Autodesk Inventor part; units mm, degrees
ref_plane "YZ Plane" through (0, 0, 0) normal (1, 0, 0) x (0, 1, 0)
ref_plane "XZ Plane" through (0, 0, 0) normal (0, 1, 0) x (-1, 0, 0)
ref_plane "XY Plane" through (0, 0, 0) normal (0, 0, 1) x (1, 0, 0)
sketch "Sketch1" plane through (0, 0, 0) normal (0, 0, 1) x (1, 0, 0)
  line L0 (0, 0) -> (0, 20) construction
  line L1 (2.5, 15) -> (97.5, 15)
  line L2 (97.5, 15) -> (97.5, -15)
  line L3 (97.5, -15) -> (2.5, -15)
  line L4 (2.5, -15) -> (2.5, 15)
  line L5 (2.5, 15) -> (97.5, -15) construction
  line L6 (97.5, 15) -> (2.5, -15) construction
  line L7 (40, 5) -> (60, 5)
  line L8 (60, 5) -> (60, -5)
  line L9 (60, -5) -> (40, -5)
  line L10 (40, -5) -> (40, 5)
  line L11 (40, 5) -> (60, -5) construction
  line L12 (60, 5) -> (40, -5) construction
  line L13 (60, 5) -> (60, 15)
  line L14 (60, -5) -> (60, -15)
  line L15 (-2.5, 15) -> (-97.5, 15)
  line L16 (-97.5, 15) -> (-97.5, -15)
  line L17 (-97.5, -15) -> (-2.5, -15)
  line L18 (-2.5, -15) -> (-2.5, 15)
  line L19 (-2.5, 15) -> (-97.5, -15) construction
  line L20 (-97.5, 15) -> (-2.5, -15) construction
  line L21 (-40, 5) -> (-60, 5)
  line L22 (-60, 5) -> (-60, -5)
  line L23 (-60, -5) -> (-40, -5)
  line L24 (-40, -5) -> (-40, 5)
  line L25 (-40, 5) -> (-60, -5) construction
  line L26 (-60, 5) -> (-40, -5) construction
  line L27 (-60, 5) -> (-60, 15)
  line L28 (-60, -5) -> (-60, -15)
  line L29 (-45, 45) -> (45, 45)
  line L30 (45, 45) -> (45, -45)
  line L31 (45, -45) -> (-45, -45)
  line L32 (-45, -45) -> (-45, 45)
  line L33 (-45, 45) -> (45, -45) construction
  line L34 (45, 45) -> (-45, -45) construction
  point P0 (50, 0)
  point P1 (50, 0)
  point P2 (-50, 0)
  point P3 (-50, 0)
  point P4 (45, 15)
  point P5 (-45, 15)
  point P6 (-45, -15)
  point P7 (45, -15)
  point P8 (45, -5)
  point P9 (45, 5)
  point P10 (-45, -5)
  point P11 (-45, 5)
  dimension "d3" = 20
  dimension "d17" = 95
  dimension "d18" = 30
  dimension "d19" = 20
  dimension "d20" = 10
  dimension "d70" = 90
  dimension "d71" = 90
  dimension "d72" = 50
extrude "Extrusion1" add sketch "Sketch1" along normal blind 5 contours L1 L2 L3 L14 L8 L13 | L30 L7 L10 L9 L3 L4 L1 | L1 L4 L3 L30 L31 L32 L17 L18 L15 L29 | L8 L9 L30 L7 | L30 L9 L10 L7 | L15 L18 L17 L32 L23 L24 L21 | L27 L22 L28 L17 L16 L15 | L32 L23 L22 L21 | L21 L24 L23 L32
sketch "Sketch2" plane through (0, 0, 5) normal (0, 0, 1) x (1, 0, 0)
  line L0 (0, 0) -> (-77.5, 0) construction
  circle A0 centre (-77.5, 0) radius 5.25
  line L1 (0, 0) -> (0, 20) construction
  circle A1 centre (-77.5, 0) radius 8
  circle A2 centre (-69.5, 0) radius 1.75
  circle A3 centre (-77.5, 8) radius 1.75
  circle A4 centre (-85.5, 0) radius 1.75
  circle A5 centre (-77.5, -8) radius 1.75
  circle A6 centre (77.5, 0) radius 5.25
  circle A7 centre (77.5, 0) radius 8
  circle A8 centre (69.5, 0) radius 1.75
  circle A9 centre (77.5, 8) radius 1.75
  circle A10 centre (85.5, 0) radius 1.75
  circle A11 centre (77.5, -8) radius 1.75
  dimension "d26" = 16
  dimension "d6" = 77.5
  dimension "d7" = 10.5
  dimension "d8" = 20
  dimension "d27" = 3.5
  dimension "d30" = 360
extrude "Extrusion2" cut sketch "Sketch2" against normal blind 7 contours A0 | A1 A2 | A1 A2 | A3 A1 | A1 A3 | A5 A1 | A1 A5 | A4 A1 | A1 A4 | A6 | A7 A10 | A7 A10 | A9 A7 | A7 A9 | A11 A7 | A7 A11 | A8 A7 | A7 A8
fillet "Fillet1" radius 3 20 edges at (-60, 5, 2.5) (-60, 15, 2.5) (-60, -5, 2.5) (-60, -15, 2.5) (-97.5, -15, 2.5) (-97.5, 15, 2.5) (97.5, 15, 2.5) (97.5, -15, 2.5) (60, -15, 2.5) (60, 15, 2.5) (60, -5, 2.5) (60, 5, 2.5) (-45, 5, 2.5) (-45, -5, 2.5) (45, 5, 2.5) (45, -5, 2.5) (-45, 45, 2.5) (45, 45, 2.5) (45, -45, 2.5) (-45, -45, 2.5)
sketch "Sketch4" plane through (0, 0, 5) normal (0, 0, 1) x (1, 0, 0)
  line L0 (-17.5, 5) -> (17.5, 5)
  line L1 (17.5, 5) -> (17.5, -5)
  line L2 (17.5, -5) -> (-17.5, -5)
  line L3 (-17.5, -5) -> (-17.5, 5)
  line L4 (-17.5, 5) -> (17.5, -5) construction
  line L5 (17.5, 5) -> (-17.5, -5) construction
  circle A0 centre (0, -5) radius 17.5
  circle A1 centre (0, 5) radius 17.5
  circle A2 centre (0, -22.5) radius 4
  circle A3 centre (0, 22.5) radius 4
  circle A4 centre (0, 0) radius 4
  circle A5 centre (16.7705, 0) radius 4
  circle A6 centre (-16.7705, 0) radius 4
  circle A7 centre (0, -12.5) radius 2.5
  circle A8 centre (0, 12.5) radius 2.5
  dimension "d32" = 35
  dimension "d33" = 10
  dimension "d34" = 35
  dimension "d35" = 35
  dimension "d36" = 8
  dimension "d37" = 8
  dimension "d38" = 8
  dimension "d39" = 8
  dimension "d40" = 8
  dimension "d41" = 5
  dimension "d42" = 5
extrude "Extrusion3" cut sketch "Sketch4" against normal blind 10 contours A6 A1 A0 L3 | L3 A6 | A3 A1 | A1 A3 | A6 A0 A1 | A8 A0 | A0 A8 | A6 A1 A0 | A1 A6 A0 | A5 A1 A0 | A0 A1 A5 | A5 L1 | L1 A5 A0 A1 | A0 A5 A1 | A2 A0 | A0 A2 | A7 A1 | A1 A7 | A4
properties part number "TAPA CUADRADA QUE DESPLAZA CON TORNILLOS"
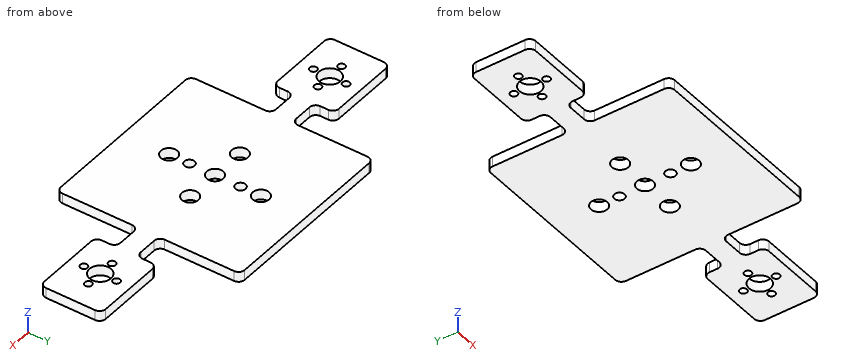
Input: part model. Units: mm. Frame: model coordinates. Give positions to 0.01 mm unless a question says otherwise; leave off trailing zeros. Order: outer loops, then holes, each group sorted by start corner. A loop starts at its lowest first (then second) coordinate and runs counter-clockwise, first axis right, second up. Notation, with made-up numbers: (-27, -1.5) - (15, -1.5) arc R11 ccw to (15, 18.5) - close; hole circle Ø9 at (-13.5, 68.25). An arc over 180 degrees is marked (long way). Write each question's results on one line, items separated by ' | '.
Item 1: Section A-A (y = 22.5). Return loops of the section in (x, z).
A:
outline: (-45, 0) - (-4, 0) - (-4, 5) - (-45, 5) - close; (4, 0) - (45, 0) - (45, 5) - (4, 5) - close
Item 2: Material intervals for line 1 along Y through (x, z) = (0, 3.55); line 2 along Y through (x, z) = (-77.5, 1.9); line 3 along X through (y, z) = (13, 1.4), sorted ascending.
A:
line 1: y = -45 to -26.5, -18.5 to -15, -10 to -4, 4 to 10, 15 to 18.5, 26.5 to 45 | line 2: y = -15 to -9.75, -6.25 to -5.25, 5.25 to 6.25, 9.75 to 15 | line 3: x = -97.33 to -60.17, -45 to -2.45, 2.45 to 45, 60.17 to 97.33
Item 3: Section C-C (x = 0). Return loops of the section in (y, z), and give its area (3 significant figures).
A:
outline: (-45, 0) - (-26.5, 0) - (-26.5, 5) - (-45, 5) - close; (-18.5, 0) - (-15, 0) - (-15, 5) - (-18.5, 5) - close; (-10, 0) - (-4, 0) - (-4, 5) - (-10, 5) - close; (4, 0) - (10, 0) - (10, 5) - (4, 5) - close; (15, 0) - (18.5, 0) - (18.5, 5) - (15, 5) - close; (26.5, 0) - (45, 0) - (45, 5) - (26.5, 5) - close | area: 280 mm^2
Item 4: Contact query for flat-ended pins moving along their axis: pin 1 Ø2 at (x, y) = (77.5, 8) entering from +Z; pin 2 Ø1.5 at (y, z) = (-21.5, 2) entering from +X; pin 3 Ø1.5 at (x, z) = (-76, 1.5) entering from +Y; pin 4 Ø2.5 at (y, z) = (-29.5, 2.5) entering from -X. Output: stop coordinate, or through.
A:
pin 1: passes through | pin 2: stops at x = 45 | pin 3: stops at y = 15 | pin 4: stops at x = -45
Item 5: Section D-D (z = 3.8). Give the number of separate pieces and of enclosed holes in the cut face, and give its area (3 significant figures).
A:
separate pieces: 1 | enclosed holes: 17 | area: 10,100 mm^2
Item 6: Section B-B (x = 85.5). Return loops of the section in (y, z).
A:
outline: (-15, 0) - (-1.75, 0) - (-1.75, 5) - (-15, 5) - close; (1.75, 0) - (15, 0) - (15, 5) - (1.75, 5) - close
